Source: three-view drawing plus pictorial views. Frame: mm from the lowest corner of the part. A direction names the side the tool comes from. Give positions to 0.01 mm unless a question says otherwise; leave off trailing zeros. Order: outer loops, then holes, each group sorted by start corner. A loop starts at its lowest first (then second) coordinate and runs counter-clockwise, first axis right, second up. Notation, with made-up numbers: (8.25, 12) - (57.25, 12) arc R9 cw to (57.25, 22) - close; hole circle Ø6 at (0, 64.5). An arc over 180 degrees is marked (long way). Answer in a Markdown table with one row per item. Add a question column.
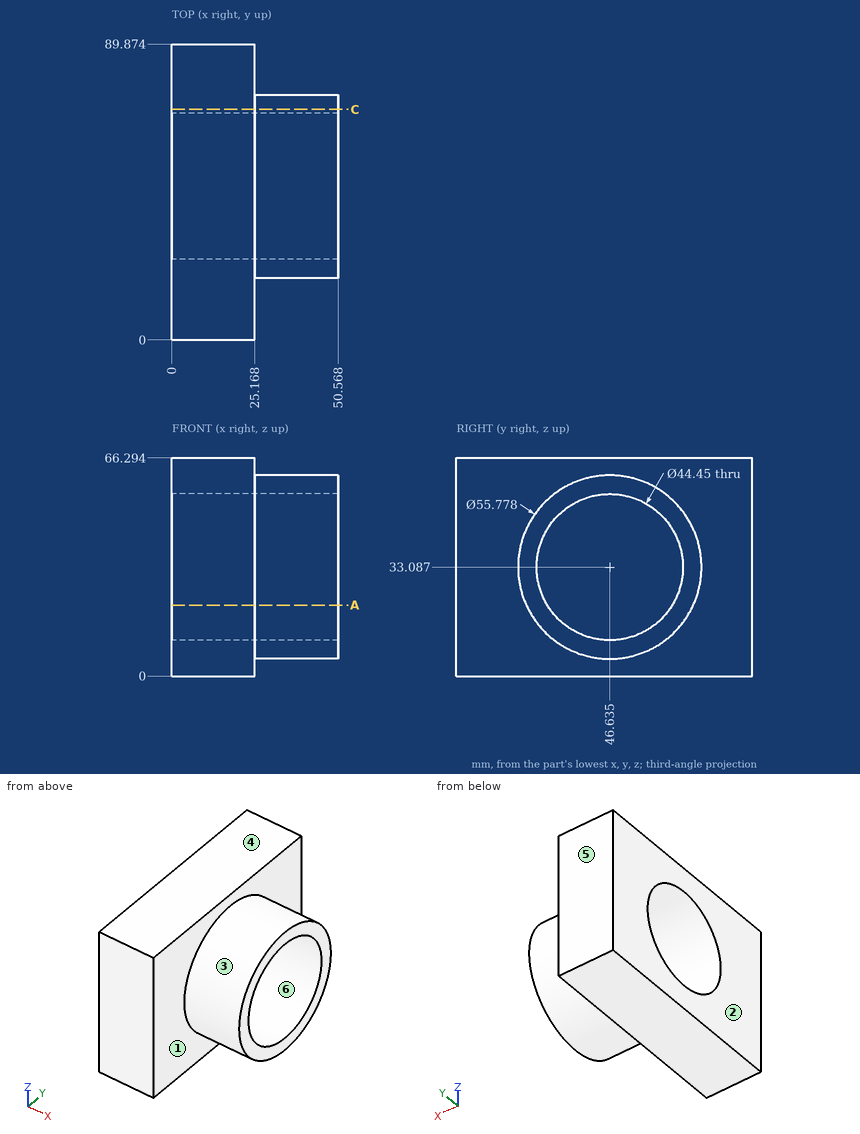
Q1. Line query: probe 1 along X at (y, z) = (74, 18); probe 2 along Y at (x, z) = (9.5, 42) (1 decimal); probe 3 along Y at (x, z) = (20, 26.5) (1 decimal). Output: solid intervals per line, ascending.
Q2. Contact query for flat-ended pins moving along their axis: P1, Ø1, axis at y = 27.5, z = 12, coming from the +X side; P2, Ø4, axis at x = 37.5, z = 41.5, coming from the -Y side; P3, Ø10, axis at x = 20.5, y = 27, coming from the -Z side. Output: stop coordinate, or through.
Q3. Section C-C, the plane y = 70. Return loops of the section in (x, z) (1 decimal), then the cut area to 3 significant figures.
Q4. Section A-A, the plane z = 21.5. Return loops of the section in (x, y) (1 decimal), then the cut area to 3 significant figures.
Q5. Access query for the marked faces 1 and 2. Directions: +Z, -Z, +X, -X, +Y, -Y. A direction counts if a zero-diameter tool reaches every point of the face in a straight line with its end or side. Return the directions, or none.
Q6. Pull-direction query (Y, two-part tool) for the marked faces 3, 4, 5 and 6; classes: +Y half, -Y half, draft (parallel to the pull), parting line (faces both ways), or undercut.
Computed:
| question | item | result |
|---|---|---|
| 1 | probe 1 | x = 0 to 25.17 |
| 1 | probe 2 | y = 0 to 26.3, 67 to 89.9 |
| 1 | probe 3 | y = 0 to 25.4, 67.9 to 89.9 |
| 2 | P1 | stops at x = 25.17 |
| 2 | P2 | stops at y = 19.49 |
| 2 | P3 | stops at z = 0 |
| 3 | outline | (0, 0) - (25.2, 0) - (25.2, 17.9) - (50.6, 17.9) - (50.6, 48.3) - (25.2, 48.3) - (25.2, 66.3) - (0, 66.3) - close |
| 3 | area | 2,440 mm^2 |
| 4 | outline | (0, 0) - (25.2, 0) - (25.2, 21.3) - (50.6, 21.3) - (50.6, 27.7) - (0, 27.7) - close; (0, 65.6) - (50.6, 65.6) - (50.6, 72) - (25.2, 72) - (25.2, 89.9) - (0, 89.9) - close |
| 4 | area | 1,630 mm^2 |
| 5 | face 1 | +X |
| 5 | face 2 | +Z, -Z, -X, +Y, -Y |
| 6 | face 3 | parting line |
| 6 | face 4 | draft |
| 6 | face 5 | +Y half |
| 6 | face 6 | undercut |
